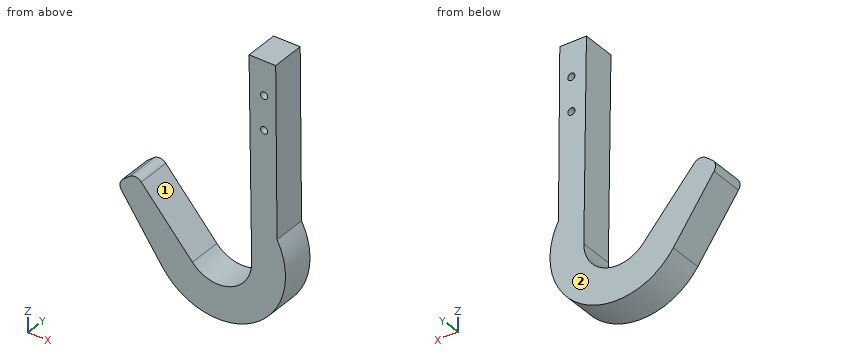
from build123d import *

# Parameters (mm, degrees)
BOSS_EXTRUDE1_DEPTH = 25.4
SKETCH2_R           = 2.667
CUT_EXTRUDE1_DEPTH  = 25.4


with BuildPart() as part:
    # Sketch1 → Boss-Extrude1 (new body)
    with BuildSketch(Plane(origin=(0, 0, 0), x_dir=(1, 0, 0), z_dir=(0, 1, 0))):
        with BuildLine():
            Line((-73.81674099, -45.828335303), (-53.81674099, -45.828335303))
            Line((-53.81674099, -45.828335303), (-52.796976786, 81.171664697))
            ThreePointArc((-52.796976786, 81.171664697), (-70.408048373, 148.917605355), (-138.959581609, 134.763114577))
            Line((-138.959581609, 134.763114577), (-169.546861653, 90.731300142))
            ThreePointArc((-169.546861653, 90.731300142), (-170.615608999, 86.194762182), (-168.299108962, 82.150479165))
            Line((-168.299108962, 82.150479165), (-163.411771612, 78.239641616))
            ThreePointArc((-163.411771612, 78.239641616), (-158.893349235, 76.871631311), (-154.679488648, 79.000239288))
            Line((-154.679488648, 79.000239288), (-116.297746729, 122.570612572))
            ThreePointArc((-116.297746729, 122.570612572), (-88.109701276, 129.483790907), (-71.840430534, 105.449049996))
            Line((-71.840430534, 105.449049996), (-73.81674099, -45.828335303))
        make_face()
    extrude(amount=BOSS_EXTRUDE1_DEPTH)

    # Sketch2 → Cut-Extrude1 (cut)
    with BuildSketch(Plane(origin=(0, 0, 0), x_dir=(-1, 0, 0), z_dir=(0, -1, 0))):
        with Locations(Location((62.503074737, 4.971664697, 0), (0, 0, 90))):
            Circle(SKETCH2_R)
        with Locations(Location((62.503074737, -20.428335303, 0), (0, 0, 90))):
            Circle(SKETCH2_R)
    extrude(amount=-CUT_EXTRUDE1_DEPTH, mode=Mode.SUBTRACT)


solid = part.part
Geometry check sheet. Reference: the model listing, model coordinates, mm. Face numbers are marked on the shaded views. A direction names the side the tool comes from. Give positions to 0.01 mm unless a question says otherwise; leave off trailing zeros. Write each loop counter-clockwise with the first axis right and the second up, starting at its lowest first coordinate (ties: lowest second). Pieces come first, ordered by that corner, then holes. Notation, with made-up numbers: (-18, 13.5) - (-7, 13.5) arc R11 ccw to (-7, 21.5) - close; hole circle Ø8 at (14, 20). An arc over 180 degrees is marked (long way). Put each result on its own line as item: value.
1. Thickness scan on line 1 (X direction, y = 19, z = -5.5); line 2 (X direction, y = 6, z = -113.5); line 3 (Z direction, x = -164, y = 7.75). Record the ranges inside material, lowest first.
Ans:
line 1: x = -73.15 to -65.12, -59.89 to -53.4
line 2: x = -153.73 to -124.29, -73.04 to -47.03
line 3: z = -98.72 to -78.71
2. Sectioned sample at B-B, the plane z = -13. Enter the section's corners in (x, y), plus the area to 3 significant figures.
Ans:
outline: (-73.05, 0) - (-53.34, 0) - (-53.34, 25.4) - (-73.05, 25.4) - close
area: 500 mm²
3. Set-up check for the marked faces 1 and 2: record each of +Z, -Z, +X, -X, +Y, -Y from which the full face is reachable in a straight line by a thin tool's end or side.
Ans:
face 1: +Z, +Y, -Y
face 2: +Z, -Z, +X, -X, +Y
4. Sectioned sample at A-A, the plane y = 15.25. Enter the section's corners in (x, z), plus the area to 3 significant figures.
Ans:
outline: (-169.55, -90.73) - (-138.96, -134.76) arc R50.8 ccw to (-52.8, -81.17) - (-53.82, 45.83) - (-73.82, 45.83) - (-71.84, -105.45) arc R25.4 cw to (-116.3, -122.57) - (-154.68, -79) arc R6.35 ccw to (-163.41, -78.24) - (-168.3, -82.15) arc R6.35 ccw to start; hole circle Ø5.33 at (-62.5, -4.97); hole circle Ø5.33 at (-62.5, 20.43)
area: 6,780 mm²
5. Sectioned sample at C-C, the plane x = -150.5. Enter the section's corners in (y, z).
Ans:
outline: (0, -118.15) - (25.4, -118.15) - (25.4, -83.74) - (0, -83.74) - close
6. Go/stop test with flat-tipped pins: pin 1 (1.5 mm diameter, centred on x = -95, y = 9.5, fed in from -Z); pin 2 (5 mm diameter, centred on y = 8, z = 4.5, fed in from +X); pin 3 (1.5 mm diameter, centred on y = 14.5, z = 17, fed in from -X). Record where each tip stops, or that it passes through.
Ans:
pin 1: stops at z = -156.56
pin 2: stops at x = -53.46
pin 3: stops at x = -73.45
